Model file for the job. Use its own axes, mm. Face numbers are marked on the shaded views. A direction names the side the tool comes from. Coordinates: 2 decimals unless noted, no trailing zeros. Write each loop counter-clockwise with the first axis right and the second up, starting at its lowest first coordinate (ties: lowest second). Pieces come first, ordered by that corner, then holes. Notation, with made-up numbers: (69.5, 47) - (84.5, 47) arc R11 ccw to (84.5, 67) - close; hole circle Ø4 at (-28.5, -24). An arc over 180 degrees is marked (long way). Put each result on its own line as item: value. Start each with the question number.
1. Saw through at B-B, the plane x = -4.5. Write the cut outline in (y, z).
2. Drop flat-ended pins along their axis: P1, Ø3, axis at y = 5, z = 12, coming from the -X side; P2, Ø19.5, axis at y = -6, z = 9.5, coming from the -X side; P3, Ø1, axis at x = -2.5, y = 22, coming from the -Z side; P4, Ø7.5, axis at y = 10, z = 10.5, coming from the +X side. Give the stop position or say it passes through.
3. Drill centre lines: L1, parallel to X at y = -17.5, z = -23; L2, parallel to Y at x = -6, z = -15; L3, parallel to Z at x = -17.5, y = 6.5. Where is each one in solid material? Low to high. Write a range as from..to.
4. Which spindle directions (+Z, -Z, +X, -X, +Y, -Y) get a long thin tool onto all of the face, cutting with end or side? Do the marked faces 4, 5 and 6. Say none if no direction does.
5. Saw through at A-A, the plane y = -24. Write the cut outline in (x, z), plus the area to 3 significant figures.
6. Saw through at C-C, the plane z = -36.5. Write the cut outline in (x, y).
7. Pull direction Z, two halves, no side cores. Call the marked faces 1, 2 and 3: released by +Z, released by -Z, zero draft, split by the parting line, or undercut.
8. Saw through at D-D, the plane y = 13.5. Give the number of separate pieces and of enclosed holes in the cut face, plus the area to 3 significant figures.
```python
from build123d import *

# Parameters (mm, degrees)
F0_W      = 52
F0_H      = 60
F1_DEPTH  = 15
F3_W      = 4
F3_H      = 9.4
F4_DEPTH  = 60
F5_DEPTH  = 56.9
F6_DEPTH  = 45
F8_DEPTH  = 63.8
F9_R      = 2.1
F10_DEPTH = 101.4
F11_START = -15
F11_DEPTH = 49.6
F13_DEPTH = 115.6
F14_R     = 0.5


with BuildPart() as f1:
    # F0 (on Top) → F1 (new body)
    with BuildSketch(Plane.XY):
        Rectangle(F0_W, F0_H)
    extrude(amount=F1_DEPTH)

    # F3 (on face) → F4 (cut, through all)
    with BuildSketch(Plane(origin=(0, 30, 0), x_dir=(-1, 0, 0), z_dir=(0, 1, 0))):
        with Locations((-24, 10.3)):
            Rectangle(F3_W, F3_H)
        with Locations((24, 10.3)):
            Rectangle(F3_W, F3_H)
    extrude(amount=-F4_DEPTH, mode=Mode.SUBTRACT)

    # F2 (on face) → F5 (cut)
    with BuildSketch(Plane(origin=(-26, 0, 0), x_dir=(0, -1, 0), z_dir=(-1, 0, 0))):
        Polygon((-21, 5.6), (-30, 15), (-30, 5.6), align=None)
        Polygon((30, 5.6), (30, 15), (21, 5.6), align=None)
    extrude(amount=-F5_DEPTH, mode=Mode.SUBTRACT)

    # F6 (add): a face of the model
    f6_faces = [f1.faces().sort_by_distance(p)[0] for p in [
        (0, 0, 0),
    ]]
    extrude(f6_faces, amount=F6_DEPTH)

    # F7 (on face) → F8 (cut)
    with BuildSketch(Plane(origin=(-26, 0, 0), x_dir=(0, -1, 0), z_dir=(-1, 0, 0))):
        Polygon((15, -45), (-30, 0), (-30, -45), align=None)
    extrude(amount=-F8_DEPTH, mode=Mode.SUBTRACT)

    # F9 (on face) → F10 (cut)
    with BuildSketch(Plane(origin=(0, 15, -15), x_dir=(1, 0, 0), z_dir=(0, 0.7071067812, -0.7071067812))):
        with Locations((-15, -4.3933982822)):
            Circle(F9_R)
        with Locations((-15, 25.6066017178)):
            Circle(F9_R)
        with Locations((15, -4.3933982822)):
            Circle(F9_R)
        with Locations((15, 25.6066017178)):
            Circle(F9_R)
    extrude(amount=-F10_DEPTH, mode=Mode.SUBTRACT)

    # F9 (on face) → F11 (cut)
    with BuildSketch(Plane(origin=(0, 15, -15), x_dir=(1, 0, 0), z_dir=(0, 0.7071067812, -0.7071067812)).offset(F11_START)):
        Polygon((-11.4, -6.4718592513), (-11.4, -2.3149373131), (-15, -0.236476344), (-18.6, -2.3149373131), (-18.6, -6.4718592513), (-15, -8.5503202204), align=None)
        with Locations((-15, -4.3933982822)):
            Circle(F9_R, mode=Mode.SUBTRACT)
        Polygon((-11.4, 23.5281407487), (-11.4, 27.6850626869), (-15, 29.763523656), (-18.6, 27.6850626869), (-18.6, 23.5281407487), (-15, 21.4496797796), align=None)
        with Locations((-15, 25.6066017178)):
            Circle(F9_R, mode=Mode.SUBTRACT)
        Polygon((11.4, 27.6850626869), (11.4, 23.5281407487), (15, 21.4496797796), (18.6, 23.5281407487), (18.6, 27.6850626869), (15, 29.763523656), align=None)
        with Locations((15, 25.6066017178)):
            Circle(F9_R, mode=Mode.SUBTRACT)
        Polygon((11.4, -2.3149373131), (11.4, -6.4718592513), (15, -8.5503202204), (18.6, -6.4718592513), (18.6, -2.3149373131), (15, -0.236476344), align=None)
        with Locations((15, -4.3933982822)):
            Circle(F9_R, mode=Mode.SUBTRACT)
    extrude(amount=-F11_DEPTH, mode=Mode.SUBTRACT)

    # F12 (on face) → F13 (cut)
    with BuildSketch(Plane(origin=(-26, 0, 0), x_dir=(0, -1, 0), z_dir=(-1, 0, 0))):
        Polygon((30, -19.7), (15, -45), (30, -45), align=None)
    extrude(amount=-F13_DEPTH, mode=Mode.SUBTRACT)

    # F14
    f14_edges = [f1.edges().sort_by_distance(p)[0] for p in [
        (0, -30, 5.6),
        (0, -30, -19.7),
        (0, 30, 5.6),
        (0, -30, 15),
        (0, 30, 15),
        (0, -21, 5.6),
        (0, 21, 5.6),
        (0, 30, 0),
        (0, -15, -45),
    ]]
    fillet(f14_edges, radius=F14_R)


solid = f1.part
```
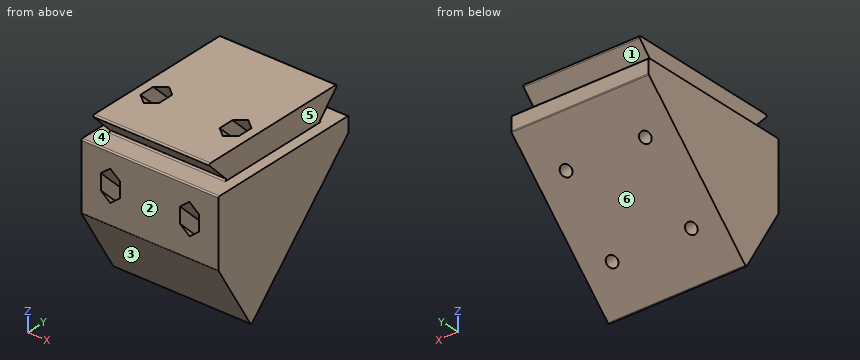
Final values:
1. outline: (-30, -19.56) arc R0.5 ccw to (-29.93, -19.82) - (-15.33, -44.45) arc R0.5 ccw to (-14.54, -44.54) - (29.85, -0.15) arc R0.5 ccw to (30, 0.21) - (30, 5.1) arc R0.5 ccw to (29.5, 5.6) - (22.17, 5.6) arc R0.5 cw to (21.81, 6.45) - (29.19, 14.15) arc R0.5 ccw to (28.83, 15) - (-28.83, 15) arc R0.5 ccw to (-29.19, 14.15) - (-21.81, 6.45) arc R0.5 cw to (-22.17, 5.6) - (-29.5, 5.6) arc R0.5 ccw to (-30, 5.1) - close
2. P1: stops at x = -22
2. P2: stops at x = -26
2. P3: stops at z = -8.5
2. P4: stops at x = 22
3. L1: x = -26..-16.95, -13.05..13.05, 16.95..26
3. L2: y = -30..15
3. L3: z = -23.5..-2.29, 3.55..15
4. face 4: none
4. face 5: +Z, +X, +Y, -Y
4. face 6: -Z, +X, -X, +Y
5. outline: (-26, -29.82) - (26, -29.82) - (26, 5.6) - (-26, 5.6) - close; (-22, 8.73) - (22, 8.73) - (22, 15) - (-22, 15) - close; hole (-18.6, -15.15) - (-15, -18.09) - (-11.4, -15.15) - (-11.4, -9.27) - (-15, -6.33) - (-18.6, -9.27) - close; hole (11.4, -15.15) - (15, -18.09) - (18.6, -15.15) - (18.6, -9.27) - (15, -6.33) - (11.4, -9.27) - close
5. area: 1,990 mm²
6. outline: (-26, -20.04) - (26, -20.04) - (26, -6.5) - (-26, -6.5) - close
7. face 1: undercut
7. face 2: zero draft
7. face 3: released by -Z
8. separate pieces: 1
8. enclosed holes: 2
8. area: 1,520 mm²
